Part model, mm, in its own coordinate system. A direction names the side the tool comes from. Coordinates: 2 decimals unless noted, no trailing zeros. Write each loop counter-clockwise with the first axis right and the second up, starting at its lowest first coordinate (ties: lowest second). Pieces come first, ordered by that corner, then holes. Notation, with made-up numbers: (-24.75, 64) -> (0.25, 64) arc R35 cw to (0.25, 100) -> close; hole circle Ø2 at (-15, -33). An arc over 180 degrees is marked (long way). One line per question, with ' | ' between items. Start each with the question number.
Item 1: Two-plate mould, pull along Y, no slides. Class faces 1 (the cylindrical face through (-0.325, 1.536, 14.07)), 2 (the cylindrical face through (2.4, 5.43, -6.07)), 3 (the flat face through (2, 0, 1)): pulls with the +Y half, pulls with the -Y half, needs draft (parallel to the pull), parting line crosses it, or undercut.
Item 2: Probe probe 1 along Z at (x, y) = (0, 2); probe 2 along X at (y, z) = (0.5, -11); probe 3 along X at (y, z) = (2.5, 0). List the from-to ranges inside material, lowest first. Write a range as [from, to].
Item 3: Saw through at C-C (y = 0.75). List the corners of the cut face in (x, z), and give its area (3 significant figures).
Item 4: Saw through at B-B (z = 16). List the corners of the cut face in (x, y).
Item 5: 3-axis set-ups, long thin cutter, end or side, ignore diameter. For faces 4 (the cylindrical face through (2.4, 5.43, 10)), 5 (the flat face through (0, 3, 9)), 6 (the cylindrical face through (-2.43, 5.4, -6.07)), 7 (the cylindrical face through (1.27, 2.96, 0.97)), 8 (the cylindrical face through (-2.43, 5.4, -14.64)): which of +Z, -Z, +X, -X, +Y, -Y reach the whole face in a straight line?
Item 6: Pin check, flat tip, straight feed: pin 1 (2.5 mm diameter, centred on x = 0, y = 3, fed in from +Z). Stop position of the tip, or through.
Item 7: Saw through at D-D (z = 4.5). List the corners of the cut face in (x, y).
Item 8: Saw through at A-A (x = 0). List the corners of the cut face in (y, z), and give its area (3 significant figures).
Autodesk Inventor part; units mm, degrees
ref_plane "YZ Plane" through (0, 0, 0) normal (1, 0, 0) x (0, 1, 0)
ref_plane "XZ Plane" through (0, 0, 0) normal (0, 1, 0) x (-1, 0, 0)
ref_plane "XY Plane" through (0, 0, 0) normal (0, 0, 1) x (1, 0, 0)
sketch "Sketch1" plane through (0, 0, 0) normal (0, 1, 0) x (-1, 0, 0)
  circle A0 centre (0, 0) radius 1.6
  circle A1 centre (0, -12) radius 1.6
  line L0 (0, 0) -> (0, 19)
  line L1 (0, 19) -> (-3, 19)
  line L2 (-3, 19) -> (-3, -18)
  line L3 (-3, -18) -> (0, -18)
  line L4 (0, -18) -> (0, 19)
  line L5 (0, 19) -> (3, 19)
  line L6 (3, 19) -> (3, -18)
  line L7 (3, -18) -> (0, -18)
  line L8 (0, -18) -> (0, 19)
  dimension "d0" = 3.2
  dimension "d1" = 3.2
  dimension "d2" = 12
  dimension "d3" = 19
  dimension "d7" = 3
  dimension "d8" = 3
extrude "Extrusion1" add sketch "Sketch1" along normal blind 6 contours A0 L0 L5 L6 L7 L4 A1 | A0 L4 A1 L3 L2 L1 L0
sketch "Sketch2" plane through (-3, 0, 19) normal (0, 0, 1) x (1, 0, 0)
  circle A0 centre (3, 3) radius 1.5
  point P0 (3, 0)
  dimension "d9" = 3
extrude "Extrusion2" cut sketch "Sketch2" against normal blind 10
fillet "Fillet1" radius 2 5 edges at (3, 3, -18) (-3, 3, -18) (0, 6, -18) (3, 6, 0.5) (-3, 6, 0.5)
properties part number "Holder Pendorong_3DPrint"
From the geometry:
1) face 1: undercut | face 2: pulls with the +Y half | face 3: pulls with the -Y half
2) probe 1: [-18, -13.6], [-10.4, -1.6], [1.6, 9] | probe 2: [-3, -1.25], [1.25, 3] | probe 3: [-3, -1.6], [1.6, 3]
3) outline: (-3, -16) arc R2 ccw to (-1, -18) -> (1, -18) arc R2 ccw to (3, -16) -> (3, 19) -> (-3, 19) -> close; hole circle Ø3.2 at (0, -12); hole circle Ø3.2 at (0, 0) | area: 204 mm2
4) outline: (-3, 0) -> (3, 0) -> (3, 4) arc R2 ccw to (1, 6) -> (-1, 6) arc R2 ccw to (-3, 4) -> close; hole circle Ø3 at (0, 3)
5) face 4: +Z, +X, +Y | face 5: +Z | face 6: -X, +Y | face 7: +Y, -Y | face 8: -Z, -X, +Y
6) pin 1: z = 9
7) outline: (-3, 0) -> (3, 0) -> (3, 4) arc R2 ccw to (1, 6) -> (-1, 6) arc R2 ccw to (-3, 4) -> close
8) outline: (0, -18) -> (4, -18) arc R2 ccw to (6, -16) -> (6, -13.6) -> (0, -13.6) -> close; (0, -10.4) -> (6, -10.4) -> (6, -1.6) -> (0, -1.6) -> close; (0, 1.6) -> (6, 1.6) -> (6, 19) -> (4.5, 19) -> (4.5, 9) -> (1.5, 9) -> (1.5, 19) -> (0, 19) -> close | area: 153 mm2
